```python
from build123d import *

# Parameters (mm, degrees)
ESQUISSE1_W             = 10.2
ESQUISSE1_H             = 5.6
BOSS_EXTRU_1_DEPTH      = 7.8
ESQUISSE2_W             = 10.2
ESQUISSE2_H             = 3.3
ENL_V_MAT_EXTRU_1_DEPTH = 0.3
ESQUISSE4_W             = 0.9
ESQUISSE4_H             = 3.3
ENL_V_MAT_EXTRU_2_DEPTH = 6.9
ESQUISSE5_W             = 5.8
ESQUISSE5_H             = 6.8
ENL_V_MAT_EXTRU_3_DEPTH = 0.7
ESQUISSE6_W             = 0.8
ESQUISSE6_H             = 0.9
ENL_V_MAT_EXTRU_4_DEPTH = 0.8
ESQUISSE7_W             = 0.8
ESQUISSE7_H             = 0.8
ENL_V_MAT_EXTRU_5_DEPTH = 0.5
ENL_V_MAT_EXTRU_6_DEPTH = 7
ENL_V_MAT_EXTRU_7_DEPTH = 0.8
ESQUISSE10_R            = 0.6
ENL_V_MAT_EXTRU_8_DEPTH = 0.5
ESQUISSE11_W            = 0.8
ESQUISSE11_H            = 0.3
ENL_V_MAT_EXTRU_9_DEPTH = 2.2


with BuildPart() as part:
    # Esquisse1 → Boss.-Extru.1 (new body)
    with BuildSketch(Plane.XY):
        Rectangle(ESQUISSE1_W, ESQUISSE1_H)
    extrude(amount=-BOSS_EXTRU_1_DEPTH)

    # Esquisse2 → Enlèv. mat.-Extru.1 (cut)
    with BuildSketch(Plane.XY):
        with Locations((0, 1.15)):
            Rectangle(ESQUISSE2_W, ESQUISSE2_H)
    extrude(amount=-ENL_V_MAT_EXTRU_1_DEPTH, mode=Mode.SUBTRACT)

    # Esquisse4 → Enlèv. mat.-Extru.2 (cut)
    with BuildSketch(Plane.XY):
        with Locations((-4.65, 1.15)):
            Rectangle(ESQUISSE4_W, ESQUISSE4_H)
        Polygon((5.1, -2.8), (5.1, -0.5), (4.2, -0.5), (4.2, -2), (-4.2, -2), (-4.2, -0.5), (-5.1, -0.5), (-5.1, -2.8), align=None)
        with Locations((4.65, 1.15)):
            Rectangle(ESQUISSE4_W, ESQUISSE4_H)
    extrude(amount=-ENL_V_MAT_EXTRU_2_DEPTH, mode=Mode.SUBTRACT)

    # Esquisse5 → Enlèv. mat.-Extru.3 (cut)
    with BuildSketch(Plane(origin=(0, 2.8, 0), x_dir=(1, 0, 0), z_dir=(0, 1, 0))):
        Polygon((-3.5, 2.91), (-3.5, 7.8), (-5.1, 7.8), (-5.1, 6.9), (-4.2, 6.9), (-4.2, 0.3), (-3.25, 0.3), (-3.85, 1.59), (-3.85, 2.56), align=None)
        Polygon((5.1, 7.8), (3.5, 7.8), (3.5, 2.91), (3.85, 2.56), (3.85, 1.59), (3.25, 0.3), (4.2, 0.3), (4.2, 6.9), (5.1, 6.9), align=None)
        with Locations((0, 3.7)):
            Rectangle(ESQUISSE5_W, ESQUISSE5_H)
    extrude(amount=-ENL_V_MAT_EXTRU_3_DEPTH, mode=Mode.SUBTRACT)

    # Esquisse6 → Enlèv. mat.-Extru.4 (cut)
    with BuildSketch(Plane.XY):
        with Locations((-2.5, -1.55)):
            Rectangle(ESQUISSE6_W, ESQUISSE6_H)
        with Locations((0, -1.55)):
            Rectangle(ESQUISSE6_W, ESQUISSE6_H)
        with Locations((2.5, -1.55)):
            Rectangle(ESQUISSE6_W, ESQUISSE6_H)
    extrude(amount=-ENL_V_MAT_EXTRU_4_DEPTH, mode=Mode.SUBTRACT)

    # Esquisse7 → Enlèv. mat.-Extru.5 (cut)
    with BuildSketch(Plane.XY.offset(-0.3)):
        with Locations((-2.5, 0.7)):
            Rectangle(ESQUISSE7_W, ESQUISSE7_H)
        with Locations((0, 0.7)):
            Rectangle(ESQUISSE7_W, ESQUISSE7_H)
        with Locations((2.5, 0.7)):
            Rectangle(ESQUISSE7_W, ESQUISSE7_H)
    extrude(amount=-ENL_V_MAT_EXTRU_5_DEPTH, mode=Mode.SUBTRACT)

    # Esquisse8 → Enlèv. mat.-Extru.6 (cut)
    with BuildSketch(Plane(origin=(0, 0, -7.8), x_dir=(-1, 0, 0), z_dir=(0, 0, -1))):
        Polygon((0.4, -1.5), (0.8, -1.5), (0.8, 1.5), (-0.8, 1.5), (-0.8, -1.5), (-0.4, -1.5), (-0.4, -1.7), (0.4, -1.7), align=None)
        with BuildLine():
            ThreePointArc((-0.7, 0.95), (-0.35, 1.3), (0, 0.95))
            ThreePointArc((0, 0.95), (0.35, 1.3), (0.7, 0.95))
            Line((0.7, 0.95), (0.7, -1.45))
            Line((0.7, -1.45), (-0.7, -1.45))
            Line((-0.7, -1.45), (-0.7, 0.95))
        make_face(mode=Mode.SUBTRACT)
        Polygon((-2.1, -1.5), (-1.7, -1.5), (-1.7, 1.5), (-3.3, 1.5), (-3.3, -1.5), (-2.9, -1.5), (-2.9, -1.7), (-2.1, -1.7), align=None)
        with BuildLine():
            ThreePointArc((-3.2, 0.95), (-2.85, 1.3), (-2.5, 0.95))
            ThreePointArc((-2.5, 0.95), (-2.15, 1.3), (-1.8, 0.95))
            Line((-1.8, 0.95), (-1.8, -1.45))
            Line((-1.8, -1.45), (-3.2, -1.45))
            Line((-3.2, -1.45), (-3.2, 0.95))
        make_face(mode=Mode.SUBTRACT)
        Polygon((2.9, -1.5), (3.3, -1.5), (3.3, 1.5), (1.7, 1.5), (1.7, -1.5), (2.1, -1.5), (2.1, -1.7), (2.9, -1.7), align=None)
        with BuildLine():
            ThreePointArc((1.8, 0.95), (2.15, 1.3), (2.5, 0.95))
            ThreePointArc((2.5, 0.95), (2.85, 1.3), (3.2, 0.95))
            Line((3.2, 0.95), (3.2, -1.45))
            Line((3.2, -1.45), (1.8, -1.45))
            Line((1.8, -1.45), (1.8, 0.95))
        make_face(mode=Mode.SUBTRACT)
    extrude(amount=-ENL_V_MAT_EXTRU_6_DEPTH, mode=Mode.SUBTRACT)

    # Esquisse9 → Enlèv. mat.-Extru.7 (cut)
    with BuildSketch(Plane(origin=(0, 0, -7.8), x_dir=(-1, 0, 0), z_dir=(0, 0, -1))):
        with BuildLine():
            Line((-0.7, 0.95), (-0.7, -1.45))
            Line((-0.7, -1.45), (0.7, -1.45))
            Line((0.7, -1.45), (0.7, 0.95))
            ThreePointArc((0.7, 0.95), (0.35, 1.3), (0, 0.95))
            ThreePointArc((0, 0.95), (-0.35, 1.3), (-0.7, 0.95))
        make_face()
        with BuildLine():
            Line((-3.2, 0.95), (-3.2, -1.45))
            Line((-3.2, -1.45), (-1.8, -1.45))
            Line((-1.8, -1.45), (-1.8, 0.95))
            ThreePointArc((-1.8, 0.95), (-2.15, 1.3), (-2.5, 0.95))
            ThreePointArc((-2.5, 0.95), (-2.85, 1.3), (-3.2, 0.95))
        make_face()
        with BuildLine():
            Line((1.8, 0.95), (1.8, -1.45))
            Line((1.8, -1.45), (3.2, -1.45))
            Line((3.2, -1.45), (3.2, 0.95))
            ThreePointArc((3.2, 0.95), (2.85, 1.3), (2.5, 0.95))
            ThreePointArc((2.5, 0.95), (2.15, 1.3), (1.8, 0.95))
        make_face()
    extrude(amount=-ENL_V_MAT_EXTRU_7_DEPTH, mode=Mode.SUBTRACT)

    # Esquisse10 → Enlèv. mat.-Extru.8 (cut)
    with BuildSketch(Plane(origin=(0, 0, -7), x_dir=(-1, 0, 0), z_dir=(0, 0, -1))):
        Circle(ESQUISSE10_R)
        with Locations((-2.5, 0)):
            Circle(ESQUISSE10_R)
        with Locations((2.5, 0)):
            Circle(ESQUISSE10_R)
    extrude(amount=-ENL_V_MAT_EXTRU_8_DEPTH, mode=Mode.SUBTRACT)

    # Esquisse11 → Enlèv. mat.-Extru.9 (cut)
    with BuildSketch(Plane.XY.offset(-0.8)):
        with Locations((-2.5, -1.85)):
            Rectangle(ESQUISSE11_W, ESQUISSE11_H)
        with Locations((0, -1.85)):
            Rectangle(ESQUISSE11_W, ESQUISSE11_H)
        with Locations((2.5, -1.85)):
            Rectangle(ESQUISSE11_W, ESQUISSE11_H)
    extrude(amount=-ENL_V_MAT_EXTRU_9_DEPTH, mode=Mode.SUBTRACT)


solid = part.part
```
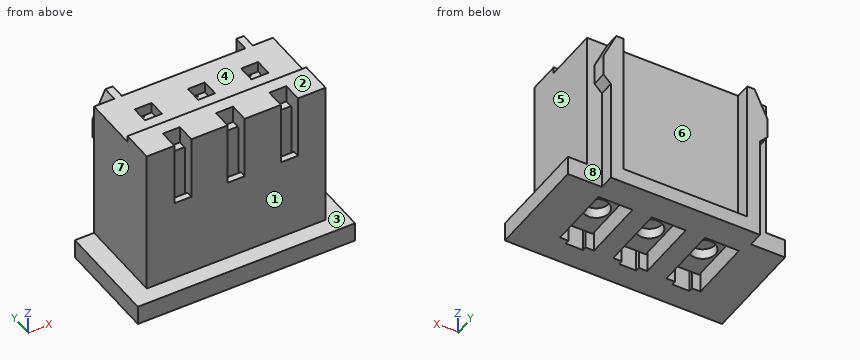
CAD build for the part. Positions are in the model's coordinates, mm. Face numbers are marked on the shaded views. A direction names the side the tool comes from. Round coordinates to 2 decimals unless told otherwise and drop trailing zeros. Order: outer loops, then holes, each group sorted by start corner. A loop starts at its lowest first (then second) coordinate and runs counter-clockwise, first axis right, second up. Notation, with made-up numbers: (80, -7) - (88, -7) arc R14 ccw to (88, 7) - close; hole circle Ø8 at (7.5, -2.75). An arc over 180 degrees is marked (long way). Answer in a Markdown table with one row per item. Add a question column.
(1) 3-axis set-ups, long thin cutter, end or side, ignore diameter. For the marked faces 1, 2, 3, 4 and 5: which of +Z, -Z, +X, -X, +Y, -Y reach the whole face in a straight line?
(2) Band-saw the part on B-B on x = -1.5. List the corners of the cut face in (y, z).
(3) Probe L1, parallel to X at y = 1.4, z = -5; L2, parallel to Y at x = 3.25, z = -4.5; L3, parallel to Z at x = 4.5, y = -2.45. List the from-to ranges inside material, lowest first. Write a range as [from, to].
(4) Mould opens along X. For the marked faces 6, 7 and 8 say: +X half, -X half, draft (parallel to the pull), parting line (faces both ways), or undercut.
(5) Band-saw the part on A-A on z = -3.5. Count the separate pieces of the cut face and the enclosed holes in it, and give its area (3 significant figures).
(6) Band-saw the part on D-D on y = -2.25. List the corners of the cut face in (x, z), and give its area (3 significant figures).
(7) Drop flat-ended pins along their axis: pin 1 Ø1.5 at (y, z) = (0, -1) entering from -X; pin 2 Ø1 at (x, y) = (-2.5, 0) entering from -Z; pin 3 Ø0.6 at (y, z) = (0.5, -0.5) entering from +X. Give the stop position or say it passes through.
Data:
| question | item | result |
|---|---|---|
| 1 | face 1 | +Z, +X, -X, -Y |
| 1 | face 2 | +Z, +X, -X, +Y, -Y |
| 1 | face 3 | +Z, -Y |
| 1 | face 4 | +Z, +X, -X, +Y |
| 1 | face 5 | +Z, +X, +Y, -Y |
| 2 | outline | (-2.8, -7.8) - (2.8, -7.8) - (2.8, -7.1) - (2.1, -7.1) - (2.1, -0.3) - (-0.5, -0.3) - (-0.5, 0) - (-2, 0) - (-2, -6.9) - (-2.8, -6.9) - close |
| 3 | L1 | x = [-4.2, -3.3], [-1.7, -0.8], [0.8, 1.7], [3.3, 4.2] |
| 3 | L2 | y = [-2, -1.5], [1.5, 2.8] |
| 3 | L3 | z = [-7.8, -6.9] |
| 4 | face 6 | undercut |
| 4 | face 7 | -X half |
| 4 | face 8 | draft |
| 5 | separate pieces | 4 |
| 5 | enclosed holes | 3 |
| 5 | area | 31.6 mm^2 |
| 6 | outline | (-5.1, -7.8) - (5.1, -7.8) - (5.1, -6.9) - (-5.1, -6.9) - close |
| 6 | area | 9.18 mm^2 |
| 7 | pin 1 | stops at x = -4.2 |
| 7 | pin 2 | stops at z = -6.5 |
| 7 | pin 3 | stops at x = 4.2 |
